from build123d import *

# Parameters (mm, degrees)
SKETCH2_R           = 8.5
BOSS_EXTRUDE1_DEPTH = 7.5


with BuildPart() as part:
    # Sketch2 → Boss-Extrude1 (new body)
    with BuildSketch(Plane(origin=(0, 0, 0), x_dir=(1, 0, 0), z_dir=(0, 1, 0))):
        with BuildLine():
            Line((-48, 61.059418618), (48, 61.059418618))
            ThreePointArc((48, 61.059418618), (67.763699658, 49.82360902), (68.217732681, 27.093868689))
            Line((68.217732681, 27.093868689), (20.217732681, -61.406131311))
            ThreePointArc((20.217732681, -61.406131311), (0, -73.440581382), (-20.217732681, -61.406131311))
            Line((-20.217732681, -61.406131311), (-68.217732681, 27.093868689))
            ThreePointArc((-68.217732681, 27.093868689), (-67.763699658, 49.82360902), (-48, 61.059418618))
        make_face()
        with Locations(Location((48, 38.059418618, 0), (0, 0, 270))):
            Circle(SKETCH2_R, mode=Mode.SUBTRACT)
        with Locations(Location((0, -50.440581382, 0), (0, 0, 270))):
            Circle(SKETCH2_R, mode=Mode.SUBTRACT)
        with Locations(Location((-48, 38.059418618, 0), (0, 0, 270))):
            Circle(SKETCH2_R, mode=Mode.SUBTRACT)
    extrude(amount=BOSS_EXTRUDE1_DEPTH)


solid = part.part
Input: part model. Units: mm. Frame: model coordinates. Give positions to 0.01 mm unless a question says otherwise; leave off trailing zeros. Order: outer loops, then holes, each group sorted by start corner. A loop starts at its lowest first (then second) coordinate and runs counter-clockwise, first axis right, second up.
Q1. Ray query, probe 1 along Z at (x, y) = (-0.5, 7.25); probe 2 along X at (y, z) = (1.75, -45); probe 3 along X at (y, z) = (6.75, -41.5). Return the intervals inside material, ascending.
Checked values:
probe 1: z = -61.06 to 41.96, 58.93 to 73.44
probe 2: x = -69.93 to -52.91, -43.09 to 43.09, 52.91 to 69.93
probe 3: x = -70.74 to -55.77, -40.23 to 40.23, 55.77 to 70.74
Q2. Section A-A on x = 0. Output: boundary loops of the cut face in (y, z), and give its area (3 significant figures).
Checked values:
outline: (0, -61.06) - (7.5, -61.06) - (7.5, 41.94) - (0, 41.94) - close; (0, 58.94) - (7.5, 58.94) - (7.5, 73.44) - (0, 73.44) - close
area: 881 mm2
Q3. Section B-B on y = 1.5. Output: boundary loops of the cut face in (x, z).
Checked values:
outline: (-68.22, -27.09) arc R23 ccw to (-48, -61.06) - (48, -61.06) arc R23 ccw to (68.22, -27.09) - (20.22, 61.41) arc R23 ccw to (-20.22, 61.41) - close; hole circle Ø17 at (-48, -38.06); hole circle Ø17 at (0, 50.44); hole circle Ø17 at (48, -38.06)
Q4. Section C-C on z = 52. Output: boundary loops of the cut face in (x, y), and give its area (3 significant figures).
Checked values:
outline: (-25.32, 0) - (-8.36, 0) - (-8.36, 7.5) - (-25.32, 7.5) - close; (8.36, 0) - (25.32, 0) - (25.32, 7.5) - (8.36, 7.5) - close
area: 254 mm2
Q5. Contact query for flat-ended pins moving along their axis: pin 1 Ø3 at (y, z) = (5, -41.5) entering from +X; pin 2 Ø2 at (y, z) = (4.5, 46) entering from -X; pin 3 Ø4 at (y, z) = (3, 8.5) entering from -X. Output: stop coordinate, or through.
Checked values:
pin 1: stops at x = 70.92
pin 2: stops at x = -29.12
pin 3: stops at x = -50
Q6. Section D-D on z = -44.5. Output: boundary loops of the cut face in (x, y), and give its area (3 significant figures).
Checked values:
outline: (-70.08, 0) - (-53.55, 0) - (-53.55, 7.5) - (-70.08, 7.5) - close; (-42.45, 0) - (42.45, 0) - (42.45, 7.5) - (-42.45, 7.5) - close; (53.55, 0) - (70.08, 0) - (70.08, 7.5) - (53.55, 7.5) - close
area: 885 mm2
Q7. Draft query along X for faces 1 (the flat face through (-43.88, 3.7, 17.78)), 2 (the cylindrical face through (-53.172, 3.698, -44.805)), 3 (the flat face through (1, 0, -10)), 4 (the flat face through (44.55, 3.7, 16.54)). Return one class per face: +X half, -X half, draft (parallel to the pull), parting line (faces both ways), or undercut.
Checked values:
face 1: -X half
face 2: undercut
face 3: draft
face 4: +X half
